```python
from build123d import *

# Parameters (mm, degrees)
SKETCH1_R   = 9.525
SKETCH1_R_2 = 8.763


with BuildPart() as part:
    # Sweep1: sweep along a path in Sketch4
    with BuildLine(Plane(origin=(0, 0, 0), x_dir=(0, 0, -1), z_dir=(1, 0, 0))) as sweep1_path:
        Line((0, 0), (0, 44.45))
        ThreePointArc((0, 44.45), (-2.434581157, 56.642978228), (-9.364958619, 66.966048107))
        Line((-9.364958619, 66.966048107), (-102.131076821, 159.192418597))
        ThreePointArc((-102.131076821, 159.192418597), (-110.447529775, 171.580102452), (-113.369027163, 186.211676326))
        Line((-113.369027163, 186.211676326), (-113.369027163, 897.411676326))
        ThreePointArc((-113.369027163, 897.411676326), (-108.254814534, 914.37875131), (-96.018442631, 927.197019796))
        Line((-96.018442631, 927.197019796), (-64.022648081, 947.882259246))
        ThreePointArc((-64.022648081, 947.882259246), (-52.338028271, 959.78322333), (-46.856249738, 975.534838814))
    # Sketch1 → Sweep1 (sweep)
    with BuildSketch(Plane(origin=(0, 0, 0), x_dir=(1, 0, 0), z_dir=(0, 1, 0))):
        Circle(SKETCH1_R)
        Circle(SKETCH1_R_2, mode=Mode.SUBTRACT)
    sweep(path=sweep1_path.line, transition=Transition.RIGHT)


solid = part.part
```
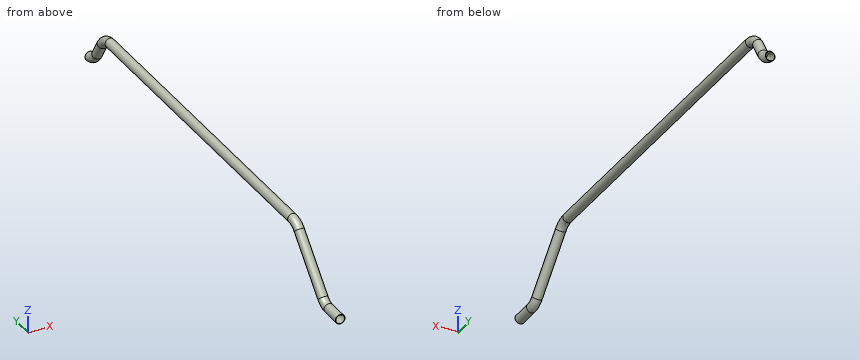
For this review, take the finished solid that the model builds, in its own axes (mm). Coordinates: 2 decimals unless noted, no trailing zeros. Write each loop counter-clockwise with the first axis right and the second up, starting at its lowest first coordinate (ties: lowest second). Pieces come first, ordered by that corner, then holes.
(1) Wall thickness on probe 1 along Z at (x, y) = (0, 20) (3 decimals); probe 2 along Y at (x, z) = (-2, 82): over which ranges is each line inside the solid? List them lowest first.
(2) Add section A-A on y = 379.5. Give the boundary of the cut face in (x, z) (3 decimals).
(3) For pin 1 Ø1 at (x, y) = (3, 170.5) entering from +Z; pin 2 Ø5 at (x, y) = (1.5, 406.5) entering from -Z; pin 3 Ø4 at (x, z) = (-1, 80.5) entering from -Y, all flat-tipped, find the tip position at first contact; note any pin that passes through.
Answer sheet:
1. probe 1: z = -9.525 to -8.763, 8.763 to 9.525
1. probe 2: y = 126.05 to 127.15, 151.21 to 152.31, 925.17 to 926.1, 946.42 to 947.35
2. outline: circle Ø19.05 at (0, 113.369); hole circle Ø17.526 at (0, 113.369)
3. pin 1: stops at z = 119.95
3. pin 2: stops at z = 103.84
3. pin 3: stops at y = 122.32
